Source: CAD feature listing. Evaluate the final solid. Frame: model axes, mm. Give positions to 0.01 mm unless a question says otherwise; leave off trailing zeros. Write each loop counter-clockwise with the first axis right and the second up, starting at its lowest first coordinate (ties: lowest second). Pieces come first, ordered by that corner, then holes.
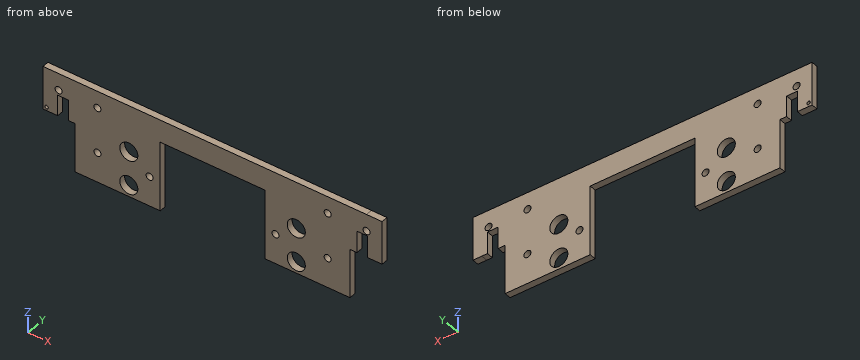
```python
from build123d import *

# Parameters (mm, degrees)
SKETCH1_R           = 0.8382
SKETCH1_R_2         = 2.159
BOSS_EXTRUDE1_DEPTH = 1.575
SKETCH2_W           = 86.242658642
SKETCH2_H           = 6.602
CUT_EXTRUDE1_DEPTH  = 65.362755899
CUT_EXTRUDE2_DEPTH  = 60.755092082
CUT_EXTRUDE3_DEPTH  = 60.755092082
SKETCH6_R           = 0.8382
CUT_EXTRUDE4_DEPTH  = 2.54
SKETCH7_W           = 65.648
SKETCH7_H           = 7.5
CUT_EXTRUDE5_DEPTH  = 58.2054366
SKETCH11_R          = 0.412551942
ID_HOLE_DEPTH       = 58.2054366
SKETCH12_W          = 2.575
SKETCH12_H          = 5
CUT_EXTRUDE6_DEPTH  = 58.2054366
SKETCH14_W          = 2.575
SKETCH14_H          = 17.002619879
CUT_EXTRUDE7_DEPTH  = 58.2054366


with BuildPart() as part:
    # Sketch1 → Boss-Extrude1 (new body)
    with BuildSketch(Plane(origin=(0, 0, 0), x_dir=(1, 0, 0), z_dir=(0, 1, 0))):
        Polygon((44.351293299, -40.014412246), (37.136293299, -40.014412246), (37.136293299, -46.615946892), (29.968293307, -46.615946892), (-30.083706693, -46.615946892), (-36.433706701, -46.615946892), (-36.433706701, -40.014412246), (-43.648706701, -40.014412246), (-43.648706701, -30.885946892), (-43.648706701, -29.647946892), (-42.378706693, -29.615946892), (-32.472706701, -29.647946892), (-32.472706701, -10.370428445), (-12.155556701, -10.370428445), (-12.155556701, -34.615947016), (-11.557706701, -34.615947016), (12.260293299, -34.615947016), (12.858143299, -34.615947016), (12.858143299, -10.370428445), (33.175293299, -10.370428445), (33.175293299, -12.929386892), (33.175293299, -29.647946892), (38.746293307, -29.615946892), (42.351293307, -29.615946892), (44.351293299, -29.615946892), (44.351293299, -31.651946892), align=None)
        with Locations(Location((-36.433706701, -35.965946892, 0), (0, 0, 270))):
            Circle(SKETCH1_R, mode=Mode.SUBTRACT)
        with Locations(Location((37.136293299, -35.983946892, 0), (0, 0, 270))):
            Circle(SKETCH1_R, mode=Mode.SUBTRACT)
        with Locations(Location((-19.648556701, -28.76738335, 0), (0, 0, 270))):
            Circle(SKETCH1_R_2, mode=Mode.SUBTRACT)
        with Locations(Location((-19.648556701, -20.63938335, 0), (0, 0, 270))):
            Circle(SKETCH1_R_2, mode=Mode.SUBTRACT)
        with Locations(Location((20.351397299, -20.63938335, 0), (0, 0, 270))):
            Circle(SKETCH1_R_2, mode=Mode.SUBTRACT)
        with Locations(Location((20.351397299, -28.76738335, 0), (0, 0, 270))):
            Circle(SKETCH1_R_2, mode=Mode.SUBTRACT)
    extrude(amount=BOSS_EXTRUDE1_DEPTH)

    # Sketch2 → Cut-Extrude1 (cut, through all)
    with BuildSketch(Plane.XZ):
        with Locations((-5.985036022, 43.314946892)):
            Rectangle(SKETCH2_W, SKETCH2_H)
    extrude(amount=-CUT_EXTRUDE1_DEPTH, mode=Mode.SUBTRACT)

    # Sketch3 → Cut-Extrude2 (cut, through all)
    with BuildSketch(Plane.XZ):
        Polygon((-40.148706701, 40.013946892), (-40.148706701, 29.623150607), (-34.773706693, 29.640513821), (-34.773706693, 8.975624969), (-46.772834391, 8.975624969), (-46.772834391, 40.013946892), align=None)
    extrude(amount=-CUT_EXTRUDE2_DEPTH, mode=Mode.SUBTRACT)

    # Sketch4 → Cut-Extrude3 (cut, through all)
    with BuildSketch(Plane.XZ):
        Polygon((40.851293299, 40.014412246), (40.851293299, 32.420104455), (40.851293299, 29.615946892), (35.476293307, 29.615946892), (35.476293307, 10.370428445), (54.710892309, 10.370428445), (54.710892309, 40.014412246), align=None)
    extrude(amount=-CUT_EXTRUDE3_DEPTH, mode=Mode.SUBTRACT)

    # Sketch6 → Cut-Extrude4 (cut)
    with BuildSketch(Plane(origin=(0, 0, 0), x_dir=(-1, 0, 0), z_dir=(0, -1, 0))):
        with Locations(Location((27.141556701, -35.947946892, 0), (0, 0, 90))):
            Circle(SKETCH6_R)
        with Locations(Location((27.141556701, -25.025946892, 0), (0, 0, 90))):
            Circle(SKETCH6_R)
        with Locations(Location((14.695556701, -25.025946892, 0), (0, 0, 90))):
            Circle(SKETCH6_R)
        with Locations(Location((-15.398143299, -25.025946892, 0), (0, 0, 90))):
            Circle(SKETCH6_R)
        with Locations(Location((-27.844397299, -25.025946892, 0), (0, 0, 90))):
            Circle(SKETCH6_R)
        with Locations(Location((-27.844397299, -35.947946892, 0), (0, 0, 90))):
            Circle(SKETCH6_R)
    extrude(amount=-CUT_EXTRUDE4_DEPTH, mode=Mode.SUBTRACT)

    # Sketch7 → Cut-Extrude5 (cut, through all)
    with BuildSketch(Plane.XZ):
        with Locations((0.351293299, 14.120428445)):
            Rectangle(SKETCH7_W, SKETCH7_H)
    extrude(amount=-CUT_EXTRUDE5_DEPTH, mode=Mode.SUBTRACT)

    # Sketch11 → ID HOLE (cut, through all)
    with BuildSketch(Plane(origin=(0, 1.575, 0), x_dir=(1, 0, 0), z_dir=(0, 1, 0))):
        with Locations(Location((-39.304798754, -30.495020326, 0), (0, 0, 270))):
            Circle(SKETCH11_R)
    extrude(amount=-ID_HOLE_DEPTH, mode=Mode.SUBTRACT)

    # Sketch12 → Cut-Extrude6 (cut, through all)
    with BuildSketch(Plane(origin=(0, 0, 0), x_dir=(-1, 0, 0), z_dir=(0, -1, 0))):
        with Locations((35.345206701, -32.134508572)):
            Rectangle(SKETCH12_W, SKETCH12_H)
    extrude(amount=-CUT_EXTRUDE6_DEPTH, mode=Mode.SUBTRACT)

    # Sketch14 → Cut-Extrude7 (cut, through all)
    with BuildSketch(Plane(origin=(0, 0, 0), x_dir=(-1, 0, 0), z_dir=(0, -1, 0))):
        with Locations((-36.109793299, -26.371738385)):
            Rectangle(SKETCH14_W, SKETCH14_H)
    extrude(amount=-CUT_EXTRUDE7_DEPTH, mode=Mode.SUBTRACT)


solid = part.part
```
1. Line query: probe 1 along X at (y, z) = (0.15, 34); probe 2 along X at (y, z) = (0.9, 28); probe 3 along Z at (x, y) = (18.5, 1.1). Output: solid intervals per line, ascending.
2. Section query C-C (x = 12). Return loops of the section in (y, z) (3 decimals).
3. Section query B-B (z = 25). Return loops of the section in (x, y) (3 decimals).
4. Pin query (flat end, axial travel): P1, Ø2.5, axis at x = 20.35, z = 28.77, coming from the -Y side; P2, Ø0.8, axis at x = 39.5, y = 1, coming from the -Z side; P3, Ø0.5, axis at y = 0.5, z = 21, coming from the +X side; P4, Ø0.8, axis at x = 5.5, y = 0.5, coming from the -Z side. Return the tip coordinate at first contact, or that it passes through.
5. Section query A-A (z = 21). Return loops of the section in (x, y) (3 decimals).
6. Section query D-D (y = 0.3). Give the number of separate pieces and of enclosed holes in the cut face, plus the area to 3 significant figures.
The answers:
1. probe 1: x = -40.15 to -36.63, -34.06 to -12.16, 12.86 to 34.82, 37.4 to 40.85
1. probe 2: x = -32.47 to -21.67, -17.63 to -12.16, 12.86 to 18.33, 22.37 to 33.18
1. probe 3: z = 17.87 to 19.53, 21.75 to 27.66, 29.88 to 40.01
2. outline: (0, 34.616) - (1.575, 34.616) - (1.575, 40.014) - (0, 40.014) - close
3. outline: (-32.473, 0) - (-27.979, 0) - (-27.979, 1.575) - (-32.473, 1.575) - close; (-26.304, 0) - (-15.533, 0) - (-15.533, 1.575) - (-26.304, 1.575) - close; (-13.858, 0) - (-12.156, 0) - (-12.156, 1.575) - (-13.858, 1.575) - close; (12.858, 0) - (14.56, 0) - (14.56, 1.575) - (12.858, 1.575) - close; (16.236, 0) - (27.007, 0) - (27.007, 1.575) - (16.236, 1.575) - close; (28.682, 0) - (33.175, 0) - (33.175, 1.575) - (28.682, 1.575) - close
4. P1: passes through
4. P2: stops at z = 29.62
4. P3: stops at x = 33.18
4. P4: stops at z = 34.62
5. outline: (-32.473, 0) - (-21.777, 0) - (-21.777, 1.575) - (-32.473, 1.575) - close; (-17.52, 0) - (-12.156, 0) - (-12.156, 1.575) - (-17.52, 1.575) - close; (12.858, 0) - (18.223, 0) - (18.223, 1.575) - (12.858, 1.575) - close; (22.48, 0) - (33.175, 0) - (33.175, 1.575) - (22.48, 1.575) - close
6. separate pieces: 1
6. enclosed holes: 13
6. area: 1,090 mm2
